```python
from build123d import *

# Parameters (mm, degrees)
SKETCH_1_W          = 15
SKETCH_1_H          = 10
SKETCH_1_W_2        = 10.5
SKETCH_1_H_2        = 7
EXTRUDE_1_DEPTH     = 650
SKETCH_2_R          = 2.15
CUT_EXTRUDE_1_DEPTH = 651.120181197
SKETCH_3_R          = 2.15
SKETCH_3_R_2        = 2.7
CUT_EXTRUDE_2_DEPTH = 651.192279253


with BuildPart() as part:
    # 草图1 → 凸台-拉伸1 (new body)
    with BuildSketch(Plane.XY):
        Rectangle(SKETCH_1_W, SKETCH_1_H)
        Rectangle(SKETCH_1_W_2, SKETCH_1_H_2, mode=Mode.SUBTRACT)
    extrude(amount=EXTRUDE_1_DEPTH)

    # 草图2 → 切除-拉伸1 (cut, through all)
    with BuildSketch(Plane.XZ.offset(5)):
        with Locations(Location((0, 640, 0), (0, 0, 270))):
            Circle(SKETCH_2_R)
        with Locations(Location((0, 625, 0), (0, 0, 270))):
            Circle(SKETCH_2_R)
        with Locations(Location((0, 610, 0), (0, 0, 270))):
            Circle(SKETCH_2_R)
        with Locations(Location((0, 10, 0), (0, 0, 270))):
            Circle(SKETCH_2_R)
        with Locations(Location((0, 25, 0), (0, 0, 270))):
            Circle(SKETCH_2_R)
        with Locations(Location((0, 40, 0), (0, 0, 270))):
            Circle(SKETCH_2_R)
    extrude(amount=-CUT_EXTRUDE_1_DEPTH, mode=Mode.SUBTRACT)

    # 草图3 → 切除-拉伸2 (cut, through all)
    with BuildSketch(Plane(origin=(7.5, 0, 0), x_dir=(0, 0, -1), z_dir=(1, 0, 0))):
        with Locations((-338, 0)):
            Circle(SKETCH_3_R)
        with Locations((-312, 0)):
            Circle(SKETCH_3_R)
        with Locations((-325, 0)):
            Circle(SKETCH_3_R_2)
    extrude(amount=-CUT_EXTRUDE_2_DEPTH, mode=Mode.SUBTRACT)


solid = part.part
```
Could you check a few things on this model? Use its own coordinates, in mm. A direction names the side the tool comes from. Round coordinates to 2 decimals unless told otherwise and drop trailing zeros. Order: outer loops, then holes, each group sorted by start corner. A loop starts at its lowest first (then second) coordinate and runs counter-clockwise, first axis right, second up. Notation, with made-up numbers: M 32.5,-0.75 L 79.5,-0.75 A12 ccw 79.5,20.25 Z; hole C 41,-27 d7. An arc over 180 degrees is marked long. One line per question, with ' | ' between items. Start each with the question number.
(1) For P1, Ø1.5, axis at x = -0.5, y = 1, coming from the +Z side, with a flat end and sliding along its axis, tell me the tip position at first contact or that it passes through.
(2) For faces 4 (the face through (0, 3.5, 320)), 5 (the face through (0, 5, 320)), which set-ups out of +Z, -Z, +X, -X, +Y, -Y let a thin tool reach every point of the face, with its end or its side?
(3) Suppose I cut it at B-B on z = 411. List the corners of the cut face in (x, y) for me.
(4) Please list where these lines run through material, in increasing order: line 1 along Y through (x, z) = (4, 380); line 2 along X through (y, z) = (1, 185); line 3 along X through (y, z) = (-4, 640).
(5) Suppose I cut it at A-A on y = 0. Count the separate pieces of the cut face and the enclosed holes in it, then the cut area to 3 significant figures.
(6) Thinking about a two-plate mould opening in X: for faces 1 (the face through (7.5, 0, 320)), 2 (the face through (0, -3.5, 320)), 3 (the face through (0, -5, 320)), which applies, +X half, -X half, draft (parallel to the pull), parting line (faces both ways), or undercut?
Geometry results:
1) P1: through
2) face 4: +Z, -Z | face 5: +Z, -Z, +X, -X, +Y
3) outline: M -7.5,-5 L 7.5,-5 L 7.5,5 L -7.5,5 Z; hole M -5.25,-3.5 L 5.25,-3.5 L 5.25,3.5 L -5.25,3.5 Z
4) line 1: -5 to -3.5, 3.5 to 5 | line 2: -7.5 to -5.25, 5.25 to 7.5 | line 3: -7.5 to -2.15, 2.15 to 7.5
5) separate pieces: 8 | enclosed holes: 0 | area: 2,860 mm²
6) face 1: +X half | face 2: undercut | face 3: draft
